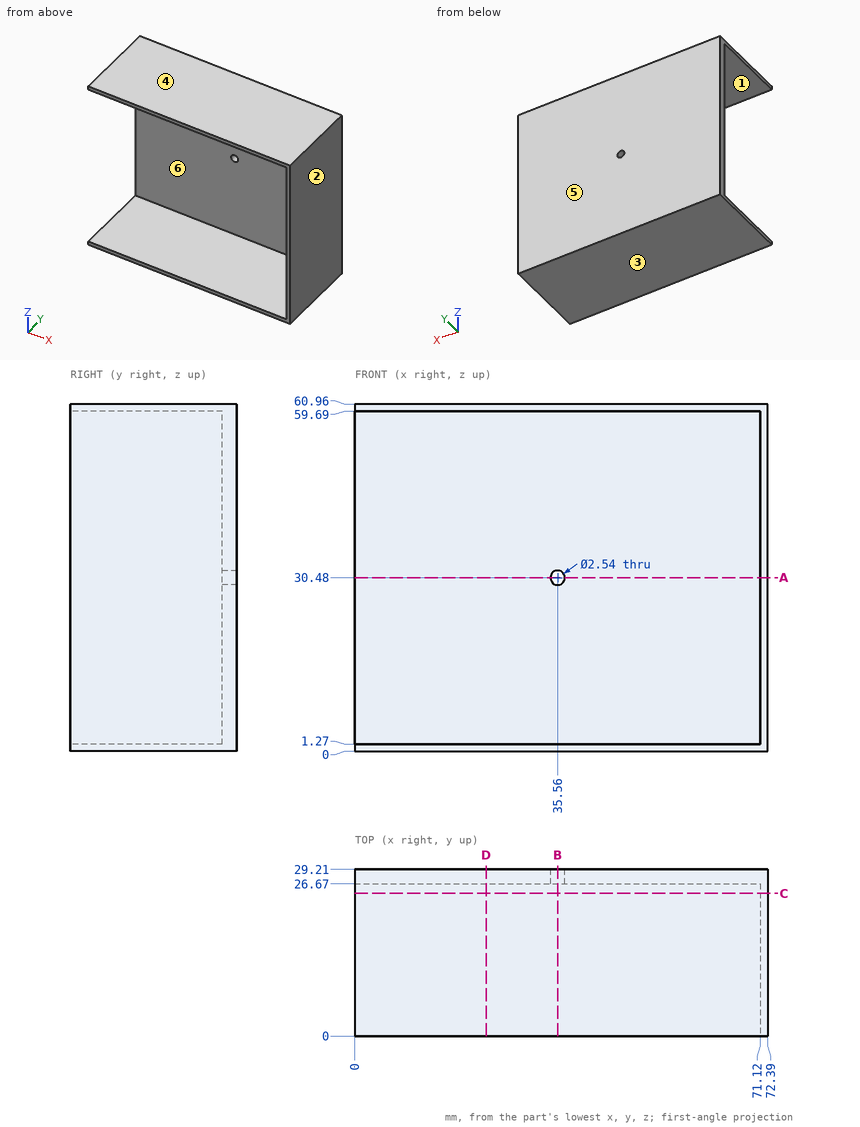
Source: three-view drawing plus pictorial views. Frame: mm from the lowest corner of the part. A direction names the side the tool comes from. Coordinates: 2 decimals unless noted, no trailing zeros. Loops run counter-clockwise (first coordinate to the right, second up) from the corner with the lowest first, then second, coordinate; pieces in that order, holes last. Notation, with made-up numbers: (28.25, 63) -> (52.25, 63) arc R25 ccw to (52.25, 98) -> close; hole circle Ø1 at (43.25, 36). An arc over 180 degrees is marked (long way). Answer in a Markdown table with one row per item. Add a question column.
Q1. Ray query, line 1 along Z through (x, y) = (40.5, 11.25); line 2 along Z through (x, y) = (35.56, 27.75); line 3 along X through (y, z) = (3.25, 28). Return the intervals inside material, ascending.
Q2. Section B-B on x = 35.56. Return the cut outline in (y, z), and give its area (3 significant figures).
Q3. Section D-D on x = 23. Return the cut outline in (y, z).
Q4. Reachability of the marked faces 5 and 6 from +Z, -Z, +X, -X, +Y, -Y: full face, straight path, thin tool, end or side. Return the list, or none.
Q5. Pull-direction query (Z, two-part tool) for the marked faces 1, 2, 3 and 4; classes: pulls with the +Z half, pulls with the -Z half, needs draft (parallel to the pull), parting line crosses it, or undercut.
Q6. Contact query for flat-ended pins moving along their axis: pin 1 Ø1.5 at (y, z) = (25, 46) entering from -X; pin 2 Ø2 at (x, z) = (38.5, 32.5) entering from -Y. Output: stop coordinate, or through.
Q7. Section A-A on z = 30.48. Return the cut outline in (x, y), and give its area (3 significant figures).
Q8. Section C-C on y = 25. Return the cut outline in (x, z).
Computed values:
| question | item | result |
|---|---|---|
| 1 | line 1 | z = 0 to 1.27, 59.69 to 60.96 |
| 1 | line 2 | z = 0 to 29.21, 31.75 to 60.96 |
| 1 | line 3 | x = 71.12 to 72.39 |
| 2 | outline | (0, 0) -> (29.21, 0) -> (29.21, 29.21) -> (26.67, 29.21) -> (26.67, 1.27) -> (0, 1.27) -> close; (0, 59.69) -> (26.67, 59.69) -> (26.67, 31.75) -> (29.21, 31.75) -> (29.21, 60.96) -> (0, 60.96) -> close |
| 2 | area | 216 mm^2 |
| 3 | outline | (0, 0) -> (29.21, 0) -> (29.21, 60.96) -> (0, 60.96) -> (0, 59.69) -> (26.67, 59.69) -> (26.67, 1.27) -> (0, 1.27) -> close |
| 4 | face 5 | +Z, -Z, +X, -X, +Y |
| 4 | face 6 | -X, -Y |
| 5 | face 1 | undercut |
| 5 | face 2 | needs draft |
| 5 | face 3 | pulls with the -Z half |
| 5 | face 4 | pulls with the +Z half |
| 6 | pin 1 | stops at x = 71.12 |
| 6 | pin 2 | stops at y = 26.67 |
| 7 | outline | (0, 26.67) -> (34.29, 26.67) -> (34.29, 29.21) -> (0, 29.21) -> close; (36.83, 26.67) -> (71.12, 26.67) -> (71.12, 0) -> (72.39, 0) -> (72.39, 29.21) -> (36.83, 29.21) -> close |
| 7 | area | 211 mm^2 |
| 8 | outline | (0, 0) -> (72.39, 0) -> (72.39, 60.96) -> (0, 60.96) -> (0, 59.69) -> (71.12, 59.69) -> (71.12, 1.27) -> (0, 1.27) -> close |
